For this review, take the finished solid that the model builds, in its own axes (mm). A direction names the side the tool comes from. Give positions to 0.01 mm unless a question says otherwise; leave off trailing zeros. Loops run counter-clockwise (first coordinate to the right, second up) from the corner with the lowest first, then second, coordinate; pieces in that order, holes last. Notation, with made-up numbers: (85, 74) -> (133, 74) arc R38 ccw to (133, 113) -> close; hole circle Ø10 at (60.25, -17). An arc over 180 degrees is marked (long way). One line per question, with ' | ' between items. Start each with the question number.
(1) Tool access review of faces 4 (the flat face through (-37.5, 0, -50)), 5 (the flat face through (17.5, 0, -40)), 6 (the flat face through (-28, 0, -35)): name each direction out of +Z, -Z, +X, -X, +Y, -Y from which nothing blocks a thin tool from reaching the whole face with its end or side.
(2) Consider section B-B (z = -29). Write out the cut boundary in (x, y), and give its area (3 significant figures).
(3) Insertion check: P1, Ø4.5, axis at x = 32.5, y = 0, coming from the -Z side; P2, Ø3, axis at y = 0, z = -41, coming from the -X side. Each pin has a flat end and moves straight along its axis. Give the tip position at first contact, or say it passes through.
(4) Consider section A-A (x = -31.5). Write out the cut boundary in (y, z), and give its area (3 significant figures).
(5) Wall thickness on probe 1 along Z at (x, y) = (33, -3); probe 2 along X at (y, z) = (2, -49); probe 3 along Y at (x, z) = (32.5, 49): over which ranges is each line inside the solid? List them lowest first.
(6) Consider section C-C (x = 22). Write out the cut boundary in (y, z).
(7) Draft analysis for pull direction X (two halves, no side actions). For faces 1 (the cylindrical face through (-29.9, -0.1, -50.1)), 2 (the flat face through (37.5, 0, 0)), 3 (the flat face through (-27, 0, 35)), state which applies: +X half, -X half, draft (parallel to the pull), parting line (faces both ways), or undercut.
from build123d import *

# Parameters (mm, degrees)
SALIENTE_EXTRUIR1_DEPTH    = 5
CORTAR_EXTRUIR1_DEPTH      = 67.755149614
CORTAR_EXTRUIR1_DEPTH_BACK = 67.755149614
CROQUIS2_R                 = 2.6


with BuildPart() as part:
    # Croquis1 → Saliente-Extruir1 (new, symmetric)
    with BuildSketch(Plane(origin=(0, 0, 0), x_dir=(1, 0, 0), z_dir=(0, 1, 0))):
        Polygon((37.5, 45), (17.5, 45), (17.5, 35), (37.5, 35), (37.5, -35), (17.5, -35), (17.5, -45), (37.5, -45), (37.5, -55), (-37.5, -55), (-37.5, -45), (-17.5, -45), (-17.5, -35), (-37.5, -35), (-37.5, 35), (-17.5, 35), (-17.5, 45), (-37.5, 45), (-37.5, 55), (37.5, 55), align=None)
    extrude(amount=SALIENTE_EXTRUIR1_DEPTH, both=True)

    # Croquis2 → Cortar-Extruir1 (cut, two sides: drawn at the far end of the back side and taken through both)
    with BuildSketch(Plane.XY.offset(-CORTAR_EXTRUIR1_DEPTH_BACK)):
        with Locations((32.5, 0)):
            Circle(CROQUIS2_R)
        with Locations(Location((-32.5, 0, 0), (0, 0, 180))):
            Circle(CROQUIS2_R)
    extrude(amount=CORTAR_EXTRUIR1_DEPTH + CORTAR_EXTRUIR1_DEPTH_BACK, mode=Mode.SUBTRACT)


solid = part.part
A:
1) face 4: +Z, -Z, -X, +Y, -Y | face 5: +X, +Y, -Y | face 6: -X, +Y, -Y
2) outline: (-37.5, -5) -> (37.5, -5) -> (37.5, 5) -> (-37.5, 5) -> close; hole circle Ø5.2 at (-32.5, 0); hole circle Ø5.2 at (32.5, 0) | area: 708 mm^2
3) P1: passes through | P2: stops at x = -17.5
4) outline: (-5, -55) -> (-2.4, -55) -> (-2.4, -45) -> (-5, -45) -> close; (-5, -35) -> (-2.4, -35) -> (-2.4, 35) -> (-5, 35) -> close; (-5, 45) -> (-2.4, 45) -> (-2.4, 55) -> (-5, 55) -> close; (2.4, -55) -> (5, -55) -> (5, -45) -> (2.4, -45) -> close; (2.4, -35) -> (5, -35) -> (5, 35) -> (2.4, 35) -> close; (2.4, 45) -> (5, 45) -> (5, 55) -> (2.4, 55) -> close | area: 468 mm^2
5) probe 1: z = -55 to -45, -35 to 35, 45 to 55 | probe 2: x = -37.5 to -34.16, -30.84 to 30.84, 34.16 to 37.5 | probe 3: y = -5 to -2.6, 2.6 to 5
6) outline: (-5, -55) -> (5, -55) -> (5, -45) -> (-5, -45) -> close; (-5, -35) -> (5, -35) -> (5, 35) -> (-5, 35) -> close; (-5, 45) -> (5, 45) -> (5, 55) -> (-5, 55) -> close
7) face 1: undercut | face 2: +X half | face 3: draft
